Autodesk Inventor part; units mm, degrees
ref_plane "Work Plane1" through (0, 7, 0) normal (0, 1, 0) x (-1, 0, 0)
ref_plane "YZ Plane" through (0, 0, 0) normal (1, 0, 0) x (0, 1, 0)
ref_plane "XY Plane" through (0, 0, 0) normal (0, 0, 1) x (1, 0, 0)
sketch "Sketch1" plane through (0, 0, 0) normal (0, 1, 0) x (-1, 0, 0)
  line L0 (0, 0) -> (0, -6.25)
  line L1 (0, 0) -> (-1, 0)
  line L2 (-1, 0) -> (-1, 0.75)
  line L3 (0, -6.25) -> (-1, -6.25)
  line L4 (-1, 0.75) -> (-15, 0.75)
  line L5 (-15, 0.75) -> (-15, -6.25)
  line L6 (-15, -6.25) -> (-1, -6.25)
  line L7 (-15, -6.25) -> (-15, -1.5)
  line L8 (-15, -6.25) -> (-15, -0.05)
  line L9 (-15, 0.75) -> (-15, -0.05)
  line L10 (-15, -0.05) -> (-11.0162, -1.5)
  line L11 (-11.0162, -1.5) -> (-4, -1.5)
  line L12 (-4, -1.5) -> (-1, -6.25)
  line L13 (-11.0162, -1.5) -> (-4, -1.5)
  dimension "d0" = 6.25
  dimension "d3" = 0.75
  dimension "d5" = 4.75
  dimension "d6" = 6.2
  dimension "d7" = 0.8
  dimension "d11" = 11
revolve "Revolution1" add sketch "Sketch1" angle 360 about axis through (0, 0, -6.25) along (1, 0, 0) contours L0 L3 L12 L11 L10 L5 L4 L2 L1
sketch "Sketch2" plane through (0, 0, 0) normal (0, 0, 1) x (1, 0, 0)
  point P0 (0, 0)
ref_plane "Work Plane1" through (0, 7, 0) normal (0, 1, 0) x (-1, 0, 0)
sketch "Sketch3" plane through (0, 7, 0) normal (0, 1, 0) x (-1, 0, 0)
  line L0 (-15, -12.45) -> (-15, -0.05)
  line L1 (-15, -6.25) -> (-7.5, -6.25)
  circle A0 centre (-7.5, -6.25) radius 1.5
  point P0 (0, 0)
  dimension "d14" = 7.5
  dimension "d15" = 3
hole "Hole1" at (7.5, 7, -6.25) direction (0, -1, 0) diameter 3 end through all
properties part number "KOLBEN PART 11" material "Brass, Soft Yellow"
Design review of the part built by this model. Coordinates are the model's own, in mm. A direction names the side the tool comes from. Coordinates: 2 decimals unless noted, no trailing zeros. Loops run counter-clockwise (first coordinate to the right, second up) from the corner with the lowest first, then second, coordinate; pieces in that order, holes last.
Q1. The part is to be moulded in two halves that separate along Y. For faces 1 (the face through (1.52, -0.04, -7.07)), 2 (the face through (8.1, 6.2, -3)), 3 (the face through (7.43, -5.77, -7.75)), say which applies: +Y half, -Y half, draft (parallel to the pull), parting line (faces both ways), or undercut.
Reported:
face 1: undercut
face 2: parting line
face 3: draft
Q2. We need section B-B on x = 12.5. State the section outline as (y, z) points, and give its area (3 significant figures).
Reported:
outline: circle Ø14 at (0, -6.25); hole circle Ø10.58 at (0, -6.25)
area: 66.0 mm2
Q3. For pin 1 (1.8 mm diameter, centred on x = 7.5, z = -6.25, fed in from +Y); pin 2 (6 mm diameter, centred on y = 1, z = -11.5, fed in from -X); pin 3 (1.5 mm diameter, centred on x = 10.5, y = 2.5, fed in from -Z); pin 4 (8 mm diameter, centred on x = 7.5, z = -1.5, fed in from -Y), all flat-tipped, find the tip position at first contact; note any pin that passes through.
Reported:
pin 1: passes through
pin 2: stops at x = 0
pin 3: stops at z = -13.03
pin 4: stops at y = -6.94
Q4. To check wall thickness, follow line 1 (Y direction, x = 9.5, z = -6.25); line 2 (X direction, y = -4.5, z = -1.25); line 3 (Y direction, x = 2, z = -3). State the ranges of each line that lie inside material, in increasing order.
Reported:
line 1: y = -7 to -4.75, 4.75 to 7
line 2: x = 1 to 15
line 3: y = -6.2 to 6.2
Q5. We need section A-A on x = 7.5. State the section outline as (y, z) points.
Reported:
outline: (-6.84, -7.75) arc R7 ccw to (6.84, -7.75) - (4.51, -7.75) arc R4.75 cw to (-4.51, -7.75) - close; (-6.84, -4.75) - (-4.51, -4.75) arc R4.75 cw to (4.51, -4.75) - (6.84, -4.75) arc R7 ccw to start
Q6. Tool access review of faces 4 (the face through (0.51, -4.22, -10.86)), 5 (the face through (8.075, 5.736, -4.864)), 6 (the face through (7.459, -1.819, -1.862)): name each direction out of +Z, -Z, +X, -X, +Y, -Y from which nothing blocks a thin tool from reaching the whole face with its end or side.
Reported:
face 4: -X
face 5: +Y, -Y
face 6: +X
